from build123d import *

# Parameters (mm, degrees)
F0_W     = 152.4
F0_H     = 279.4
F1_DEPTH = 53.975
F2_R     = 10.779843
F2_R_2   = 11.914255
F2_W     = 11.361208
F2_H     = 29.29996
F2_W_2   = 11.959181
F2_H_2   = 30.495897
F2_R_3   = 10.911721
F2_R_4   = 12.092973
F2_R_5   = 13.276833
F2_R_6   = 13.27683
F2_R_7   = 7.22516
F2_R_8   = 7.657603
F2_R_9   = 9.282801
F2_R_10  = 8.96937
F2_R_11  = 11.282249
F3_DEPTH = 12.7


with BuildPart() as f1:
    # F0 (on Front) → F1 (new body)
    with BuildSketch(Plane.XZ):
        with Locations((76.2, 139.7)):
            Rectangle(F0_W, F0_H)
    extrude(amount=-F1_DEPTH)

    # F2 (on face) → F3 (join)
    with BuildSketch(Plane.XZ):
        Polygon((48.956591, 64.652771), (22.718993, 64.652771), (9.600193, 41.930344), (22.718993, 19.207917), (48.956591, 19.207917), (62.07539, 41.930344), align=None)
        with Locations((32.250043, 136.407822)):
            Circle(F2_R)
        with Locations((32.250043, 190.224111)):
            Circle(F2_R_2)
        with Locations((34.342894, 258.092411)):
            Rectangle(F2_W, F2_H)
        with Locations((73.509186, 258.092425)):
            Rectangle(F2_W_2, F2_H_2)
        with Locations((81.28266, 191.420019)):
            Circle(F2_R_3)
        with Locations((80.08673, 136.407822)):
            Circle(F2_R_4)
        with Locations((80.684699, 94.550714)):
            Circle(F2_R_5)
        with Locations((118.954055, 39.53851)):
            Circle(F2_R_6)
        with Locations((77.694908, 43.126259)):
            Circle(F2_R_7)
        with Locations((124.335676, 93.952753)):
            Circle(F2_R_8)
        with Locations((124.933645, 135.2119)):
            Circle(F2_R_9)
        with Locations((126.727521, 191.420019)):
            Circle(F2_R_10)
        with Locations((124.933645, 245.236307)):
            Circle(F2_R_11)
    extrude(amount=F3_DEPTH)


solid = f1.part
Geometry check sheet. Reference: the model listing, model coordinates, mm. A direction names the side the tool comes from. Round coordinates to 2 decimals unless told otherwise and drop trailing zeros. Order: outer loops, then holes, each group sorted by start corner. A loop starts at its lowest first (then second) coordinate and runs counter-clockwise, first axis right, second up. Notation, with made-up numbers: M 16,30 L 24,30 A21 ccw 24,59 Z; hole C 77.25,50 d7. An arc over 180 degrees is marked long. Answer in a Markdown table with one row per item.
(1) Tool access check on faces 4 (the face through (30.699, -6.261, 202.037)), 5 (the face through (34, -6, 272.742)), 6 (the face through (36, -6, 19.208)). Record the directions out of +Z, -Z, +X, -X, +Y, -Y that give a thin tool (end or side, any length) a straight path to the whole face; none if there is none.
Responses:
| item | result |
|---|---|
| face 4 | -Y |
| face 5 | +Z, -X, -Y |
| face 6 | -Z, +X, -X, -Y |
(2) Go/stop test with flat-tipped pins: P1, Ø6.5, axis at y = -4.5, z = 261.5, coming from the +X side; P2, Ø3.5, axis at x = 36, y = -9.5, coming from the -Z side; P3, Ø6, axis at x = 72, y = -4, coming from the +Z side. Record where each tip stops, or that it passes through.
Responses:
| item | result |
|---|---|
| P1 | stops at x = 79.49 |
| P2 | stops at z = 19.21 |
| P3 | stops at z = 273.34 |
(3) Sectioned sample at A-A, the plane y = -4.5. State how many separate pieces and enclosed holes the cut face has, and give its area (3 significant figures).
Responses:
| item | result |
|---|---|
| separate pieces | 14 |
| enclosed holes | 0 |
| area | 6,510 mm² |
(4) Scan lines: probe 1 along Z at (x, y) = (78, -1.5); probe 2 along X at (y, z) = (-1, 187); probe 3 along Y at (x, z) = (20, 192.5) (3 decimals). Record each from-to range of solid material in increasing order. Write a range as from..to.
Responses:
| item | result |
|---|---|
| probe 1 | z = 35.91..50.34, 81.55..107.55, 124.5..148.32, 181.01..201.83, 242.84..273.34 |
| probe 2 | x = 20.78..43.72, 71.31..91.26, 118.92..134.53 |
| probe 3 | y = 0..53.975 |
(5) Draft check along Z on faces 1 (the face through (131.549, -6.261, 198.983)), 2 (the face through (67.53, -6, 258)), 3 (the face through (55.61, -6.26, 53.13)). Enter one of: released by +Z, released by -Z, zero draft, split by the parting line, or undercut.
Responses:
| item | result |
|---|---|
| face 1 | undercut |
| face 2 | zero draft |
| face 3 | released by +Z |
(6) Sectioned sample at D-D, the plane x = 128.5. Record the cut outline in (y, z) (3 decimals), and give its area (3 significant figures).
Responses:
| item | result |
|---|---|
| outline | M -12.7,30.311 L 0,30.311 L 0,0 L 53.975,0 L 53.975,279.4 L 0,279.4 L 0,255.94 L -12.7,255.94 L -12.7,234.533 L 0,234.533 L 0,200.213 L -12.7,200.213 L -12.7,182.628 L 0,182.628 L 0,143.782 L -12.7,143.782 L -12.7,126.642 L 0,126.642 L 0,100.379 L -12.7,100.379 L -12.7,87.526 L 0,87.526 L 0,48.766 L -12.7,48.766 Z |
| area | 16,200 mm² |
(7) Sectioned sample at B-B, the plane x = 109.5. Record the cut outline in (y, z) (3 decimals), and give its area (3 significant figures).
Responses:
| item | result |
|---|---|
| outline | M -12.7,30.217 L 0,30.217 L 0,0 L 53.975,0 L 53.975,279.4 L 0,279.4 L 0,48.86 L -12.7,48.86 Z |
| area | 15,300 mm² |
(8) Sectioned sample at C-C, the plane z = 215. Record the cut outline in (x, y) (3 decimals), and give its area (3 significant figures).
Responses:
| item | result |
|---|---|
| outline | M 0,0 L 152.4,0 L 152.4,53.975 L 0,53.975 Z |
| area | 8,230 mm² |
